from build123d import *

# Parameters (mm, degrees)
SKETCH1_R           = 7
BOSS_EXTRUDE1_DEPTH = 7
BOSS_EXTRUDE1_TAPER = 10
SKETCH2_R           = 3.1
CUT_EXTRUDE1_DEPTH  = 7
SKETCH3_R           = 7
SKETCH3_R_2         = 1.65
BOSS_EXTRUDE2_DEPTH = 3
SKETCH4_R           = 2.5
SKETCH4_R_2         = 1.65
BOSS_EXTRUDE3_DEPTH = 1.8


with BuildPart() as part:
    # Sketch1 → Boss-Extrude1 (new body)
    with BuildSketch(Plane.XY):
        Circle(SKETCH1_R)
    extrude(amount=BOSS_EXTRUDE1_DEPTH, taper=BOSS_EXTRUDE1_TAPER)

    # Sketch2 → Cut-Extrude1 (cut)
    with BuildSketch(Plane.XY.offset(7)):
        Circle(SKETCH2_R)
    extrude(amount=-CUT_EXTRUDE1_DEPTH, mode=Mode.SUBTRACT)

    # Sketch3 → Boss-Extrude2 (add)
    with BuildSketch(Plane(origin=(0, 0, 0), x_dir=(-1, 0, 0), z_dir=(0, 0, -1))):
        Circle(SKETCH3_R)
        Circle(SKETCH3_R_2, mode=Mode.SUBTRACT)
    extrude(amount=BOSS_EXTRUDE2_DEPTH)

    # Sketch4 → Boss-Extrude3 (add)
    with BuildSketch(Plane(origin=(0, 0, -3), x_dir=(-1, 0, 0), z_dir=(0, 0, -1))):
        Circle(SKETCH4_R)
        Circle(SKETCH4_R_2, mode=Mode.SUBTRACT)
    extrude(amount=BOSS_EXTRUDE3_DEPTH)


solid = part.part
Model file for the job. Use its own axes, mm. A direction names the side the tool comes from. Give positions to 0.01 mm unless a question says otherwise; leave off trailing zeros. Order: outer loops, then holes, each group sorted by start corner. A loop starts at its lowest first (then second) coordinate and runs counter-clockwise, first axis right, second up. Notation, with made-up numbers: (-2.75, 64) -> (43.25, 64) arc R15 cw to (43.25, 72) -> close; hole circle Ø5 at (83, 2). An arc over 180 degrees is marked (long way). Use CSV: the item, a comma, the result in double quotes.
1. Drop flat-ended pins along their axis: pin 1 (2 mm diameter, centred on y = -3, z = 2, fed in from -X); pin 2 (3 mm diameter, centred on y = 4, z = 3.5, fed in from +X); pin 3 (3 mm diameter, centred on x = 0, y = 0, fed in from +Z); pin 4 (1 mm diameter, centred on y = 4, z = 4, fed in from +X). Give the stop position or say it passes through.
Outcome:
pin 1,"x = -6.39"
pin 2,"x = 5.93"
pin 3,"through"
pin 4,"x = 5.25"
2. 3-axis set-ups, long thin cutter, end or side, ignore diameter. For faces 5 (the flat face through (0, -3, -3)), 6 (the cylindrical face through (1.43, -2.75, 3.55)), 7 (the flat face through (-2, -1, -4.8)): which of +Z, -Z, +X, -X, +Y, -Y reach the whole face in a straight line?
Outcome:
face 5,"-Z"
face 6,"+Z"
face 7,"-Z, +X, -X, +Y, -Y"
3. Band-saw the part on A-A, the plane x = 0. Give the cut face in (y, z), then the cut area to 3 significant figures.
Outcome:
outline,"(-7, -3) -> (-2.5, -3) -> (-2.5, -4.8) -> (-1.65, -4.8) -> (-1.65, 0) -> (-3.1, 0) -> (-3.1, 7) -> (-5.77, 7) -> (-7, 0) -> close; (1.65, -4.8) -> (2.5, -4.8) -> (2.5, -3) -> (7, -3) -> (7, 0) -> (5.77, 7) -> (3.1, 7) -> (3.1, 0) -> (1.65, 0) -> close"
area,"81.1 mm²"
4. Mould opens along X. For faces 1 (the cylindrical face through (-6.466, -2.681, -1.479)), 2 (the flat face through (-1.3, -1.3, 0)), 3 (the cylindrical face through (1.216, 1.115, -2.366)), 4 (the flat face through (2.5, -2.5, 7)) say: +X half, -X half, draft (parallel to the pull), parting line (faces both ways), or undercut.
Outcome:
face 1,"parting line"
face 2,"undercut"
face 3,"undercut"
face 4,"draft"
5. Band-saw the part on C-C, the plane z = -2.5. Give the cut face in (x, y), then the cut area to 3 significant figures.
Outcome:
outline,"circle Ø14 at (0, 0); hole circle Ø3.3 at (0, 0)"
area,"145 mm²"
6. Band-saw the part on D-D, the plane z = 1.5. Give the cut face in (x, y).
Outcome:
outline,"circle Ø13.47 at (0, 0); hole circle Ø6.2 at (0, 0)"
7. Drill centre lines: line 1 along Z through (x, y) = (2.5, -2.5); line 2 along Z through (x, y) = (-2, 0.75); line 3 along Y through (x, z) = (0, -1). Where is each one in solid material? Low to high. Write a range as from..to.
Outcome:
line 1,"-3..7"
line 2,"-4.8..0"
line 3,"-7..-1.65, 1.65..7"
